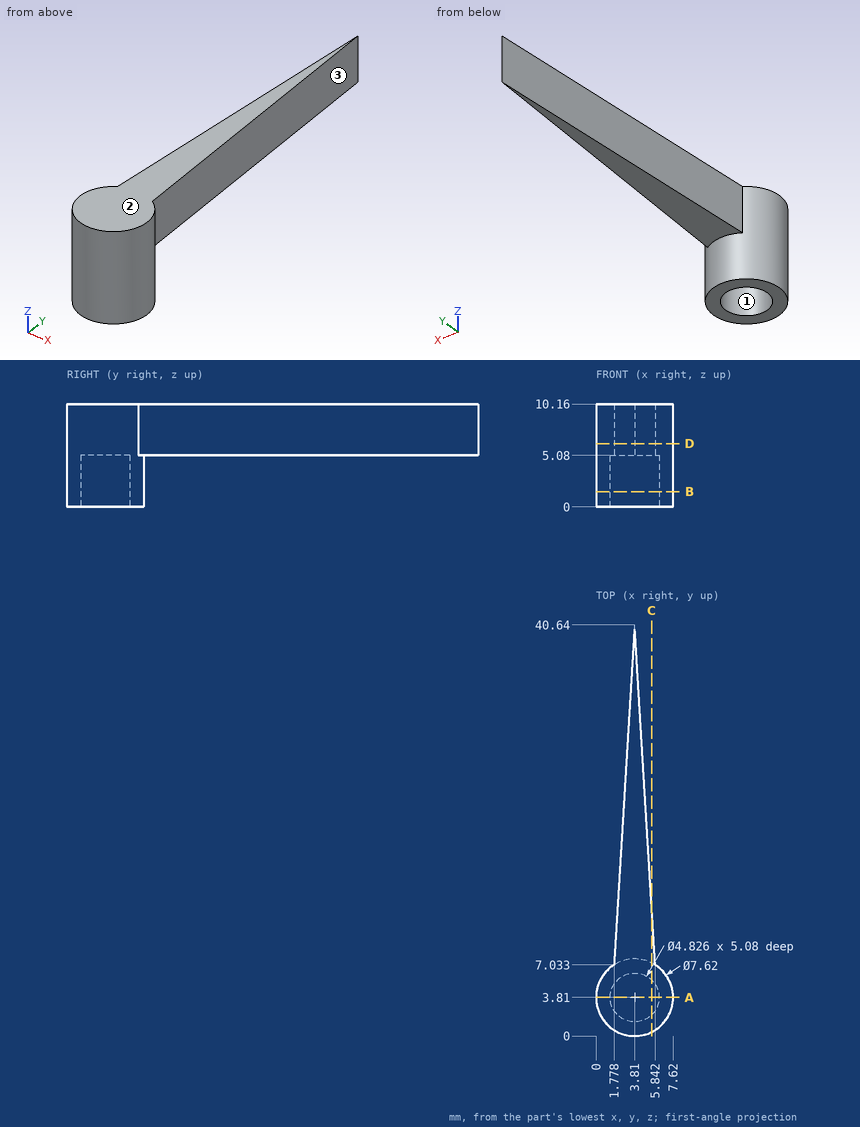
Study the drawing (mm; zero at the part's minimum x, y, z) and answer. Coordinates: 2 decimals unless noted, no trailing zeros. Order: outer loops, then holes, each group sorted by start corner. A loop starts at its lowest first (then second) coordinate and runs counter-clockwise, first axis right, second up. Notation, with made-up numbers: M 85,67 L 105,67 A25 ccw 105,97 Z; hole C -1.5,39 d6. An arc over 180 degrees is marked long. Answer as a JSON object with one key per item and string values. Group by question number.
1. Determine the mould class of the marked faces 1, 2 and 3 for opening direction X: released by +X, released by -X, zero draft, split by the parting line, or undercut.
2. Section D-D on z = 6.25 is taken. Write down the section's boundary in (x, y), then the cut area to 3 significant figures.
3. Section C-C on x = 5.5 is taken. Write down the section's boundary in (y, z) (1 decimal).
4. Section B-B on z = 1.5 is taken. Write down the section's boundary in (x, y).
5. Straight lines are drawn through the part: line 1 (Y direction, x = 4, z = 4) (1 decimal); line 2 (Z direction, x = 3.5, y = 19); line 3 (X direction, y = 3, z = 2). For each, find the intervals that lie inside material, in ascending order.
6. Flat-ended cylindrical pins translate along their axes: P1, Ø3, axis at y = 6.5, z = 4.5, coming from the +X side; P2, Ø6, axis at y = 27.5, z = 5.5, coming from the -X side; P3, Ø4, axis at y = 35.5, z = 7.5, coming from the -X side; P4, Ø2, axis at x = 3, z = 4.5, coming from the -Y side. Find the tip coordinate at first contact, or state that the pin passes through.
7. Section A-A on y = 3.81 is taken. Write down the section's boundary in (x, z), then the cut area to 3 significant figures.
Values follow:
{
 "1": {"face 1": "undercut", "face 2": "zero draft", "face 3": "released by +X"},
 "2": {"outline": "M 1.78,7.03 A3.81 ccw long 5.84,7.03 L 3.81,40.64 Z", "area": "112 mm2"},
 "3": {"outline": "M 0.4,0 L 2.1,0 L 2.1,5.1 L 5.5,5.1 L 5.5,0 L 7.2,0 L 7.2,5.1 L 12.7,5.1 L 12.7,10.2 L 0.4,10.2 Z"},
 "4": {"outline": "C 3.81,3.81 d7.62; hole C 3.81,3.81 d4.83"},
 "5": {"line 1": "0 to 1.4, 6.2 to 7.6", "line 2": "5.08 to 10.16", "line 3": "0.09 to 1.54, 6.08 to 7.53"},
 "6": {"P1": "x = 7.43", "P2": "x = 2.83", "P3": "x = 3.38", "P4": "y = 0"},
 "7": {"outline": "M 0,0 L 1.4,0 L 1.4,5.08 L 6.22,5.08 L 6.22,0 L 7.62,0 L 7.62,10.16 L 0,10.16 Z", "area": "52.9 mm2"}
}
